Read the model definition and answer for the solid it produces. Units are mm, in the model's axes. Face numbers are marked on the shaded views. A direction names the side the tool comes from. Round coordinates to 2 decimals unless told otherwise and drop trailing zeros. Loops run counter-clockwise (first coordinate to the right, second up) from the corner with the lowest first, then second, coordinate; pieces in that order, holes last. Notation, with made-up numbers: M 7.25,-11.5 L 50.25,-11.5 A27 ccw 50.25,4.5 Z; hole C 44.25,-39.75 d1. An arc over 180 degrees is marked long. Write each question's results on one line, items separated by ' | '.
from build123d import *

# Parameters (mm, degrees)
BOSS_EXTRUDE1_DEPTH = 120
SKETCH4_R           = 3.3
CUT_EXTRUDE1_DEPTH  = 201.688813839
SKETCH5_R           = 2.75
CUT_EXTRUDE2_DEPTH  = 202.285866369


with BuildPart() as part:
    # Sketch2 → Boss-Extrude1 (new body)
    with BuildSketch(Plane.XY):
        Polygon((0, 0), (0, 100), (4, 100), (4, 4), (130, 4), (130, 0), align=None)
    extrude(amount=BOSS_EXTRUDE1_DEPTH)

    # Sketch4 → Cut-Extrude1 (cut, through all)
    with BuildSketch(Plane(origin=(4, 0, 0), x_dir=(0, 0, -1), z_dir=(1, 0, 0))):
        with Locations(Location((-100, 80, 0), (0, 0, 90))):
            Circle(SKETCH4_R)
        with Locations(Location((-20, 80, 0), (0, 0, 90))):
            Circle(SKETCH4_R)
        with Locations(Location((-20, 20, 0), (0, 0, 90))):
            Circle(SKETCH4_R)
        with Locations(Location((-100, 20, 0), (0, 0, 90))):
            Circle(SKETCH4_R)
    extrude(amount=-CUT_EXTRUDE1_DEPTH, mode=Mode.SUBTRACT)

    # Sketch5 → Cut-Extrude2 (cut, through all)
    with BuildSketch(Plane(origin=(0, 4, 0), x_dir=(1, 0, 0), z_dir=(0, 1, 0))):
        with Locations(Location((100, -30, 0), (0, 0, 180))):
            Circle(SKETCH5_R)
        with Locations(Location((50, -30, 0), (0, 0, 180))):
            Circle(SKETCH5_R)
        with Locations(Location((50, -90, 0), (0, 0, 180))):
            Circle(SKETCH5_R)
        with Locations(Location((100, -90, 0), (0, 0, 180))):
            Circle(SKETCH5_R)
    extrude(amount=-CUT_EXTRUDE2_DEPTH, mode=Mode.SUBTRACT)


solid = part.part
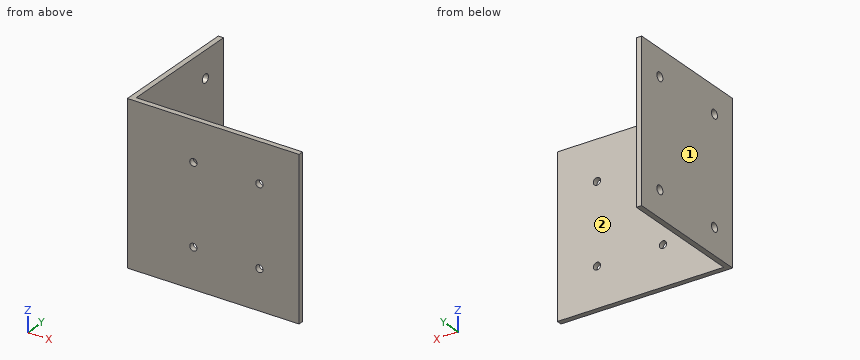
Item 1: The part is cut by section D-D (y = 70.5). Determine the outline of the cut face in (x, z).
Outcome:
outline: M 0,0 L 4,0 L 4,120 L 0,120 Z
Item 2: Straight lines are drawn through the part: line 1 (Z direction, x = 100, y = 1.35); line 2 (Z direction, x = 2, y = 80); line 3 (Y direction, x = 46, z = 30). For each, find the intervals that lie inside material, in ascending order.
Outcome:
line 1: z = 0 to 27.25, 32.75 to 87.25, 92.75 to 120 | line 2: z = 0 to 16.7, 23.3 to 96.7, 103.3 to 120 | line 3: y = 0 to 4
Item 3: For the marked faces 1 and 2, determine the directions among +Z, -Z, +X, -X, +Y, -Y from which every point of the face is accessible in a straight line to the end or side of a thin tool.
Outcome:
face 1: +Z, -Z, -X, +Y, -Y | face 2: +Z, -Z, +X, +Y
Item 4: Flat-ended cylindrical pins translate along their axes: pin 1 (9 mm diameter, centred on x = 50, z = 90, fed in from -Y); pin 2 (8.5 mm diameter, centred on y = 80, z = 100, fed in from +X); pin 3 (2 mm diameter, centred on x = 47.5, z = 84, fed in from +Y). Find the tip coordinate at first contact, or state that the pin passes through.
Outcome:
pin 1: stops at y = 0 | pin 2: stops at x = 4 | pin 3: stops at y = 4
Item 5: The part is cut by section C-C (x = 50). Determine the outline of the cut face in (y, z).
Outcome:
outline: M 0,0 L 4,0 L 4,27.25 L 0,27.25 Z; M 0,32.75 L 4,32.75 L 4,87.25 L 0,87.25 Z; M 0,92.75 L 4,92.75 L 4,120 L 0,120 Z
Item 6: The part is cut by section B-B (y = 20). Determine the outline of the cut face in (x, z), plus the area to 3 significant figures.
Outcome:
outline: M 0,0 L 4,0 L 4,16.7 L 0,16.7 Z; M 0,23.3 L 4,23.3 L 4,96.7 L 0,96.7 Z; M 0,103.3 L 4,103.3 L 4,120 L 0,120 Z | area: 427 mm2
Item 7: The part is cut by section A-A (z = 30). Determine the outline of the cut face in (x, y).
Outcome:
outline: M 0,0 L 47.25,0 L 47.25,4 L 4,4 L 4,100 L 0,100 Z; M 52.75,0 L 97.25,0 L 97.25,4 L 52.75,4 Z; M 102.75,0 L 130,0 L 130,4 L 102.75,4 Z
